Read the model definition and answer for the solid it produces. Units are mm, in the model's axes. Face numbers are marked on the shaded views. A direction names the side the tool comes from. Coordinates: 2 decimals unless noted, no trailing zeros. Loops run counter-clockwise (first coordinate to the right, second up) from the corner with the lowest first, then second, coordinate; pieces in that order, holes last. Notation, with made-up numbers: (-10, 0) -> (15, 0) arc R17 ccw to (15, 4) -> close; hole circle Ø1 at (51, 44.5). An arc over 180 degrees is marked (long way). Answer as a JSON object with one key per item and string values. Group by question number.
Q1. Each of these flat-tipped pins is pushed along its axis until it touches: P1, Ø5, axis at y = 9.5, z = 8, coming from the +X side; P2, Ø12, axis at y = 11, z = 10, coming from the +X side; P3, Ø3.5, axis at x = 16, z = 10, coming from the +Y side. Where does it stop, or does it pass through?
Q2. The part is cut by section D-D on z = 9.5. State how many separate pieces and enclosed holes the cut face has, and give its area (3 significant figures).
Q3. The part is cut by section B-B on x = 32.5. Write down the section's boundary in (y, z).
Q4. For the marked faces 1 and 2, determine the directions among +Z, -Z, +X, -X, +Y, -Y from which every point of the face is accessible in a straight line to the end or side of a thin tool.
Q5. Straight lines are drawn through the part: line 1 along Z through (x, y) = (16, 63); line 2 along Z through (x, y) = (16, 4.75); line 3 along Z through (x, y) = (10.5, 10.5). For each, find the intervals that lie inside material, in ascending order. Write a range as [from, to].
Q6. Determine the mould class of the marked faces 3, 4, 5 and 6 for opening direction X: released by +X, released by -X, zero draft, split by the parting line, or undercut.
Q7. The part is cut by section A-A on y = 10.5. Write down the section's boundary in (x, z).
Q8. The part is cut by section C-C on y = 19.5. Write down the section's boundary in (x, z), and give its area (3 significant figures).
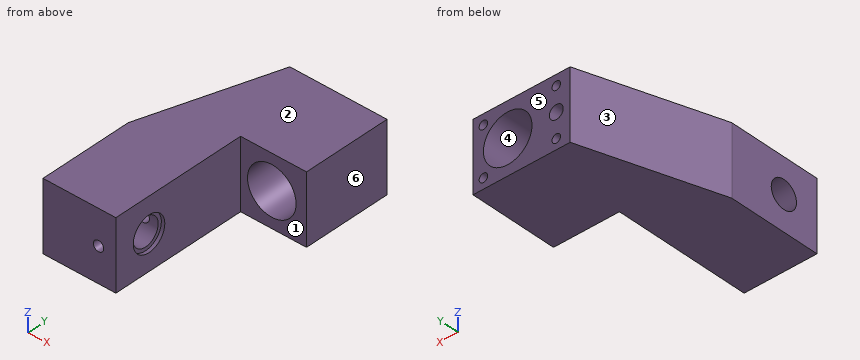
Autodesk Inventor part; units mm, degrees
ref_plane "Arbeitsebene1" through (0, 12, 0) normal (0, 1, 0) x (-1, 0, 0)
ref_plane "Arbeitsebene2" through (26.5, 0, 0) normal (1, 0, 0) x (0, 1, 0)
ref_plane "XY Plane" through (0, 0, 0) normal (0, 0, 1) x (1, 0, 0)
sketch "Skizze1" plane through (0, 0, 0) normal (0, 0, 1) x (1, 0, 0)
  line L0 (0, 0) -> (0, 27)
  line L1 (0, 27) -> (12, 65)
  line L2 (12, 65) -> (40, 65)
  line L3 (40, 65) -> (40, 39.5)
  line L4 (40, 39.5) -> (21, 39.5)
  line L5 (21, 39.5) -> (21, 0)
  line L6 (21, 0) -> (0, 0)
  dimension "d0" = 65
  dimension "d1" = 21
  dimension "d2" = 39.5
  dimension "d3" = 38
  dimension "d4" = 28
  dimension "d5" = 12
extrude "Extrusion1" add sketch "Skizze1" along normal blind 20
sketch "Skizze3" plane through (12, 65, 0) normal (0, 1, 0) x (1, 0, 0)
  line L0 (0, 0) -> (0, -20)
  line L1 (28, 0) -> (28, -20)
  point P0 (-12, 0)
  point P1 (18, -10)
  point P2 (28, -10)
  dimension "d16" = 10
hole "Bohrung2" at (30, 65, 10) direction (0, -1, 0) diameter 14 end through all
sketch "Skizze4" plane through (12, 65, 0) normal (0, 1, 0) x (1, 0, 0)
  line L0 (0, 0) -> (0, -20)
  line L1 (28, 0) -> (28, -20)
  point P0 (-12, 0)
  point P1 (4, -10)
  point P2 (28, -10)
  dimension "d24" = 4
hole "Bohrung3" at (16, 65, 10) direction (0, -1, 0) diameter 3 depth 65 counterbore diameter 4 counterbore depth 30
sketch "Skizze5" plane through (21, 0, 0) normal (1, 0, 0) x (0, 0, -1)
  line L0 (0, 0) -> (-20, 0)
  point P0 (-10, 10.5)
  point P1 (-10, 0)
  dimension "d32" = 10.5
hole "Bohrung4" at (21, 10.5, 10) direction (-1, 0, 0) diameter 8 depth 21 counterbore diameter 10 counterbore depth 1
ref_plane "Arbeitsebene1" through (0, 12, 0) normal (0, 1, 0) x (-1, 0, 0)
sketch "Skizze8" plane through (12, 65, 0) normal (0, 1, 0) x (1, 0, 0)
  circle A0 centre (4, -10) radius 2
  circle A1 centre (18, -10) radius 7
  line L0 (28, 0) -> (0, 0)
  line L1 (0, 0) -> (0, -20)
  line L2 (28, -20) -> (0, -20)
  line L3 (28, 0) -> (28, -20)
  line L4 (4, -10) -> (4, -3) construction
  line L5 (4, -10) -> (4, -17) construction
  line L6 (18, -10) -> (9, -10) construction
  line L7 (9, 0) -> (9, -20)
  point P0 (-12, 0)
  dimension "d57" = 14
hole "Bohrung7" at (16, 65, 17) at (16, 65, 3) direction (0, -1, 0) diameter 2.459 depth 9 tip angle 118
ref_plane "Arbeitsebene2" through (26.5, 0, 0) normal (1, 0, 0) x (0, 1, 0)
mirror "Spiegeln2" about plane through (26.5, 0, 0) normal (1, 0, 0) of "Bohrung7"
properties part number "MotorBlock" material "Stahl, galvanisiert"
Final values:
{
 "1": {"P1": "stops at x = 20", "P2": "stops at x = 21", "P3": "stops at y = 35"},
 "2": {"separate pieces": "5", "enclosed holes": "0", "area": "904 mm2"},
 "3": {"outline": "(39.5, 0) -> (65, 0) -> (65, 3.46) -> (39.5, 3.46) -> close; (39.5, 16.54) -> (65, 16.54) -> (65, 20) -> (39.5, 20) -> close"},
 "4": {"face 1": "+Z, -Z, +X, -Y", "face 2": "+Z, +X, -X, +Y, -Y"},
 "5": {"line 1": "z = [0, 1.77], [4.23, 8], [12, 15.77], [18.23, 20]", "line 2": "z = [0, 8.5], [11.5, 20]", "line 3": "z = [0, 6], [14, 20]"},
 "6": {"face 3": "released by -X", "face 4": "undercut", "face 5": "zero draft", "face 6": "released by +X"},
 "7": {"outline": "(0, 0) -> (21, 0) -> (21, 5) -> (20, 5) -> (20, 6) -> (0, 6) -> close; (0, 14) -> (20, 14) -> (20, 15) -> (21, 15) -> (21, 20) -> (0, 20) -> close"},
 "8": {"outline": "(0, 0) -> (21, 0) -> (21, 20) -> (0, 20) -> close; hole circle Ø3 at (16, 10)", "area": "413 mm2"}
}
